from build123d import *

# Parameters (mm, degrees)
ESQUISSE1_W             = 10.15
ESQUISSE1_H             = 15.5
EXTRUSION1_DEPTH        = 1.1
ESQUISSE2_R             = 1.875
ENL_V_MAT_EXTRU_1_DEPTH = 19.560239761
CHANFREIN1_SIZE         = 2
ESQUISSE3_W             = 10.15
ESQUISSE3_H             = 8
EXTRUSION2_DEPTH        = 3.3
ESQUISSE5_R             = 0.5
ESQUISSE9_R             = 0.5


with BuildPart() as part:
    # Esquisse1 → Extrusion1 (new body)
    with BuildSketch(Plane.XY):
        with Locations((5.075, 7.75)):
            Rectangle(ESQUISSE1_W, ESQUISSE1_H)
    extrude(amount=EXTRUSION1_DEPTH)

    # Esquisse2 → Enlèv. mat.-Extru.1 (cut, through all)
    with BuildSketch(Plane.XY.offset(1.1)):
        with Locations((5.075, 12.85)):
            Circle(ESQUISSE2_R)
    extrude(amount=-ENL_V_MAT_EXTRU_1_DEPTH, mode=Mode.SUBTRACT)

    # Chanfrein1
    chanfrein1_edges = [part.edges().sort_by_distance(p)[0] for p in [
        (0, 15.5, 0.55),
        (10.15, 15.5, 0.55),
    ]]
    chamfer(chanfrein1_edges, length=CHANFREIN1_SIZE)

    # Esquisse3 → Extrusion2 (add)
    with BuildSketch(Plane.XY.offset(1.1)):
        with Locations((5.075, 4)):
            Rectangle(ESQUISSE3_W, ESQUISSE3_H)
    extrude(amount=EXTRUSION2_DEPTH)

    # Balayage1: sweep along a path in Esquisse8
    with BuildLine(Plane(origin=(2.54, 0, 0), x_dir=(0, 0, -1), z_dir=(1, 0, 0))) as balayage1_path:
        Line((-2.25, 0), (-2.25, -3.05))
        ThreePointArc((-2.25, -3.05), (-1.957106781, -3.757106781), (-1.25, -4.05))
        Line((-1.25, -4.05), (0.791981695, -4.05))
    # Esquisse5 → Balayage1 (sweep)
    with BuildSketch(Plane.XZ):
        with Locations((2.535, 2.2)):
            Circle(ESQUISSE5_R)
    balayage1 = sweep(path=balayage1_path.line)

    # Balayage2: sweep along a path in Esquisse10
    with BuildLine(Plane(origin=(5.08, 0, 0), x_dir=(0, 0, -1), z_dir=(1, 0, 0))) as balayage2_path:
        Line((-2.25, 0), (-2.25, -3.05))
        ThreePointArc((-2.25, -3.05), (-1.957106781, -3.757106781), (-1.25, -4.05))
        Line((-1.25, -4.05), (0.791981695, -4.05))
    # Esquisse9 → Balayage2 (sweep)
    with BuildSketch(Plane.XZ):
        with Locations((5.075, 2.25)):
            Circle(ESQUISSE9_R)
    sweep(path=balayage2_path.line)

    # Symétrie1: Balayage1 across plane
    add(balayage1.mirror(Plane(origin=(5.08, 0, 0), x_dir=(0, 0, 1), z_dir=(1, 0, 0))))


solid = part.part
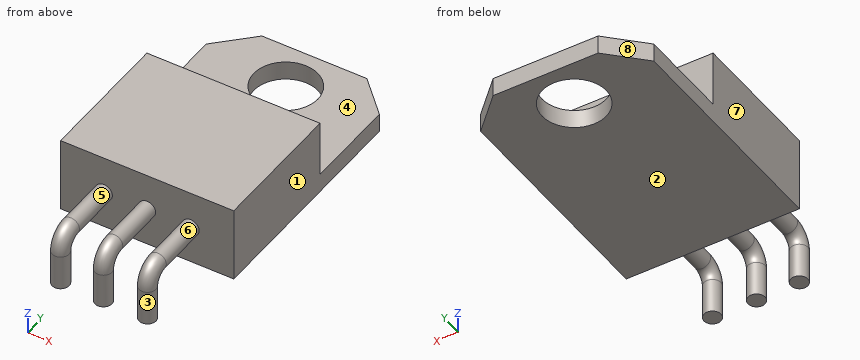
Work out the finished part from the listing and answer in its coordinate system (mm). Face numbers are marked on the shaded views. A direction names the side the tool comes from. Round coordinates to 2 decimals unless told otherwise and drop trailing zeros. Loops run counter-clockwise (first coordinate to the right, second up) from the corner with the lowest first, then second, coordinate; pieces in that order, holes last. Notation, with made-up numbers: (26.5, -25) - (46.5, -25) arc R11 ccw to (46.5, -12) - close; hole circle Ø3 at (-4, -26). An arc over 180 degrees is marked (long way). One line per item, written item: value.
Q1. Find section D-D on y = 4.25. Give the vertices of the cut face in (x, z), and give its area (3 significant figures).
Check values:
outline: (0, 0) - (10.15, 0) - (10.15, 4.4) - (0, 4.4) - close
area: 44.7 mm2
Q2. For the marked faces 1, 2, 3, 4 and 5, determine the directions among +Z, -Z, +X, -X, +Y, -Y from which every point of the face is accessible in a straight line to the end or side of a thin tool.
Check values:
face 1: +Z, -Z, +X, +Y, -Y
face 2: -Z, +X, -X, +Y
face 3: -Z
face 4: +Z, +X, -X, +Y
face 5: none
Q3. Find section B-B on y = 12.85. Give the vertices of the cut face in (x, z).
Check values:
outline: (0, 0) - (3.2, 0) - (3.2, 1.1) - (0, 1.1) - close; (6.95, 0) - (10.15, 0) - (10.15, 1.1) - (6.95, 1.1) - close
Q4. Find section A-A on z = 0.7. Give the vertices of the cut face in (x, y) (3 decimals), and give its area (3 significant figures).
Check values:
outline: (0, 0) - (10.15, 0) - (10.15, 13.5) - (8.15, 15.5) - (2, 15.5) - (0, 13.5) - close; circle Ø1 at (2.535, -4); circle Ø1 at (5.075, -4.05); circle Ø1 at (7.625, -4); hole circle Ø3.75 at (5.075, 12.85)
area: 145 mm2
Q5. Find section C-C on x = 0.5. Give the vertices of the cut face in (y, z).
Check values:
outline: (0, 0) - (14, 0) - (14, 1.1) - (8, 1.1) - (8, 4.4) - (0, 4.4) - close
Q6. Straight lines are drawn through the part: probe 1 along X at (y, z) = (-3.25, 2.5); probe 2 along Y at (x, z) = (7, 1.45); probe 3 along Z at (x, y) = (8, 2). For each, find the intervals that lie inside material, in ascending order.
Check values:
probe 1: 2.15 to 2.92, 4.65 to 5.5, 7.24 to 8.01
probe 2: 0 to 8
probe 3: 0 to 4.4
Q7. Each of these flat-tipped pins is pushed along its axis until it touches: pin 1 Ø2 at (x, z) = (2.5, 4) entering from +Y; pin 2 Ø1.5 at (x, y) = (1, 12) entering from -Z; pin 3 Ø2 at (x, y) = (7.5, 11) entering from +Z. Where does it stop, or does it pass through?
Check values:
pin 1: y = 8
pin 2: z = 0
pin 3: z = 1.1
Q8. The mould has two halves that part along Y. Classify the marked faces 6, 7 and 8: +Y half, -Y half, draft (parallel to the pull), parting line (faces both ways), or undercut.
Check values:
face 6: undercut
face 7: draft
face 8: +Y half
